Can you work these out from the model? Positions are in its coordinate system, mm. Give positions to 0.01 mm unless a question says otherwise; leave off trailing zeros. Write each loop counter-clockwise with the first axis right and the second up, starting at its lowest first coordinate (ties: lowest second). Pieces come first, ordered by that corner, then holes. Notation, with made-up numbers: (63.5, 5) -> (81.5, 5) arc R14 ccw to (81.5, 9) -> close; hole circle Ø10 at (40.5, 85.5). An arc over 180 degrees is marked (long way). One line per item, written item: value.
from build123d import *

# Parameters (mm, degrees)
SKETCH1_W                                      = 32
SKETCH1_H                                      = 32
EXTRUDE2_DEPTH                                 = 7
CSK_FOR_M6_FLAT_HEAD_MACHINE_SCREW1_AT_2_COUNT = 2
CSK_FOR_M6_FLAT_HEAD_MACHINE_SCREW1_AT_2_PITCH = 16


with BuildPart() as part:
    # Sketch1 → Extrude2 (new body)
    with BuildSketch(Plane.XY):
        with Locations((16, 16)):
            Rectangle(SKETCH1_W, SKETCH1_H)
    extrude(amount=EXTRUDE2_DEPTH)

    # Sketch2 → CSK for M6 Flat Head Machine Screw1 (revolve, cut)
    with BuildSketch(Plane(origin=(8, 16, 7), x_dir=(0, -1, 0), z_dir=(1, 0, 0))):
        Polygon((0, 0), (0, 7), (3.3, 7), (3.3, 5.196152423), (6.3, 0), align=None)
    csk_for_m6_flat_head_machine_screw1 = revolve(axis=Axis((8, 16, 13.35), (0, 0, -1)), mode=Mode.SUBTRACT)

    # CSK for M6 Flat Head Machine Screw1 at 2: CSK for M6 Flat Head Machine Screw1 ×2
    with Locations(*[(i * CSK_FOR_M6_FLAT_HEAD_MACHINE_SCREW1_AT_2_PITCH, 0, 0) for i in range(1, CSK_FOR_M6_FLAT_HEAD_MACHINE_SCREW1_AT_2_COUNT)]):
        add(csk_for_m6_flat_head_machine_screw1, mode=Mode.SUBTRACT)


solid = part.part
1) I need wall thicknesses on L1, parallel to X at y = 16, z = 1; L2, parallel to Y at x = 24, z = 1.15; L3, parallel to X at y = 12, z = 6. Which ranges of each line are inside material? Lowest first, please.
Answer list:
L1: x = 0 to 4.7, 11.3 to 20.7, 27.3 to 32
L2: y = 0 to 12.7, 19.3 to 32
L3: x = 0 to 3.91, 12.09 to 19.91, 28.09 to 32
2) Will this pin go through, and if not, where does the flat tip stop? pin 1 (7.5 mm diameter, centred on x = 8, y = 16, fed in from +Z).
Answer list:
pin 1: stops at z = 2.58
3) If we section it at A-A (x = 8): Write out the boundary of the cut face in (y, z).
Answer list:
outline: (0, 0) -> (12.7, 0) -> (12.7, 1.8) -> (9.7, 7) -> (0, 7) -> close; (19.3, 0) -> (32, 0) -> (32, 7) -> (22.3, 7) -> (19.3, 1.8) -> close
4) If we section it at C-C (z = 3): Write out the boundary of the cut face in (x, y), and give its area (3 significant figures).
Answer list:
outline: (0, 0) -> (32, 0) -> (32, 32) -> (0, 32) -> close; hole circle Ø7.98 at (8, 16); hole circle Ø7.98 at (24, 16)
area: 924 mm^2
5) We'd pull the mould along X, two halves only. Please class faces 1 (the face through (0, 16, 3)), 2 (the face through (16, 16, 0)), 3 (the face through (27.22, 16.72, 0.91)): released by +X, released by -X, zero draft, split by the parting line, or undercut.
Answer list:
face 1: released by -X
face 2: zero draft
face 3: undercut
6) If we section it at D-D (z = 5.75): Write out the boundary of the cut face in (x, y).
Answer list:
outline: (0, 0) -> (32, 0) -> (32, 32) -> (0, 32) -> close; hole circle Ø11.16 at (8, 16); hole circle Ø11.16 at (24, 16)
7) If we section it at B-B (y = 16): Write out the boundary of the cut face in (x, z), and give its area (3 significant figures).
Answer list:
outline: (0, 0) -> (4.7, 0) -> (4.7, 1.8) -> (1.7, 7) -> (0, 7) -> close; (11.3, 0) -> (20.7, 0) -> (20.7, 1.8) -> (17.7, 7) -> (14.3, 7) -> (11.3, 1.8) -> close; (27.3, 0) -> (32, 0) -> (32, 7) -> (30.3, 7) -> (27.3, 1.8) -> close
area: 100 mm^2
